Input: dimensioned drawing with shaded views. Units: mm. Origin: part minimum x, y, z. Round coordinates to 2 decimals unless told otherwise and drop trailing zeros. Write each loop counter-clockwise with the first axis right and the second up, starting at its lowest first coordinate (ties: lowest second). Pieces come first, ordered by that corner, then holes. Notation, with made-up numbers: (-23.5, -17) - (17.5, -17) arc R28 cw to (17.5, 11) - close; hole circle Ø8 at (27, 24). An arc over 180 degrees is marked (long way). Use one line per item in the form item = value.
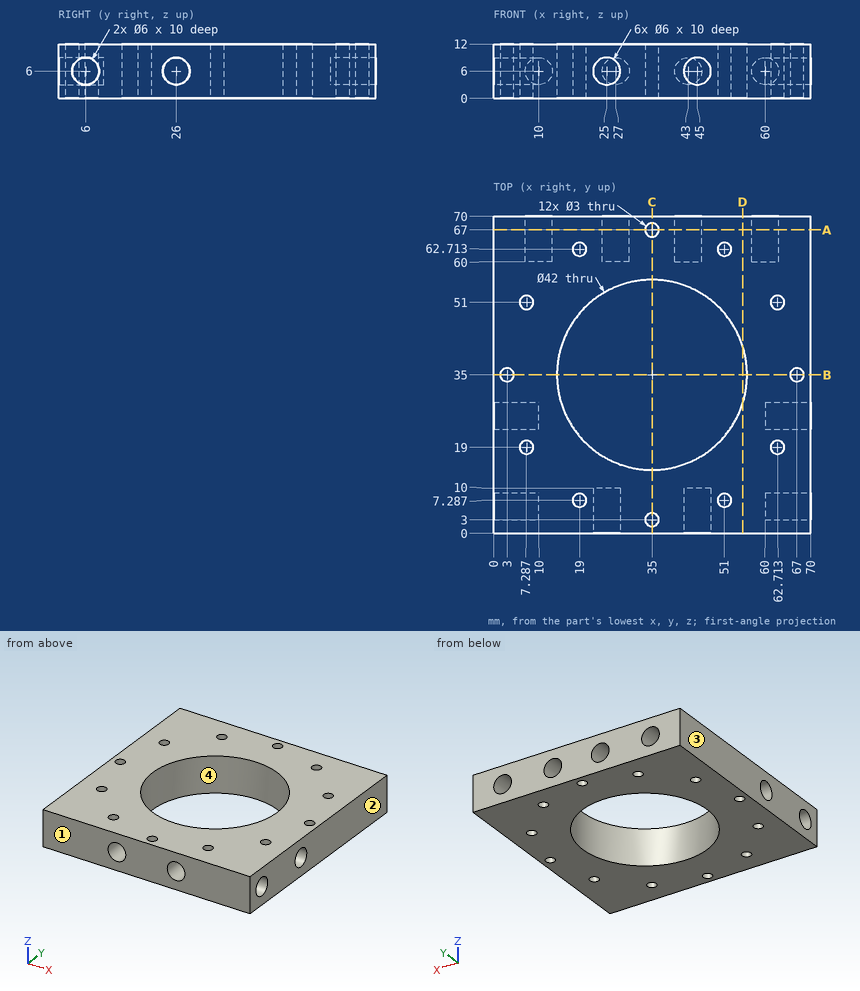
(1) Draft query along X for the marked faces 1, 2, 3 and 4. Return one class per face: released by +X, released by -X, zero draft, split by the parting line, or undercut.
Derived:
face_1 = zero draft
face_2 = released by +X
face_3 = released by -X
face_4 = undercut
(2) Cut plane D-D on x = 55. Output: boundary loops of the cut face in (y, z), then the cut area to 3 significant figures.
Derived:
outline = (0, 0) - (28.6, 0) - (28.6, 12) - (0, 12) - close; (41.4, 0) - (70, 0) - (70, 12) - (41.4, 12) - close
area = 686 mm^2
(3) Cut plane A-A on y = 67. Output: boundary loops of the cut face in (x, z), then the cut area to 3 significant figures.
Derived:
outline = (0, 0) - (33.5, 0) - (33.5, 12) - (0, 12) - close; (36.5, 0) - (70, 0) - (70, 12) - (36.5, 12) - close; hole circle Ø6 at (10, 6); hole circle Ø6 at (27, 6); hole circle Ø6 at (43, 6); hole circle Ø6 at (60, 6)
area = 691 mm^2
(4) Cut plane B-B on y = 35. Output: boundary loops of the cut face in (x, z), then the cut area to 3 significant figures.
Derived:
outline = (0, 0) - (1.5, 0) - (1.5, 12) - (0, 12) - close; (4.5, 0) - (14, 0) - (14, 12) - (4.5, 12) - close; (56, 0) - (65.5, 0) - (65.5, 12) - (56, 12) - close; (68.5, 0) - (70, 0) - (70, 12) - (68.5, 12) - close
area = 264 mm^2
(5) First-contact query: pin 1 Ø2.5 at (x, y) = (51, 7.29) entering from -Z; pin 2 Ø1.5 at (x, z) = (59, 7.5) entering from +Y; pin 3 Ø3 at (y, z) = (25, 7) entering from +X. Flat tips, straight axial feed; report the tip coordinate or a pass-through.
Derived:
pin_1 = through
pin_2 = 60
pin_3 = 60
(6) Material intervals for L1, parallel to X at y = 5.5, z = 5.75; L2, parallel to Y at x = 51, z = 9.25; L3, parallel to X at y = 67.25, z = 6, sorted ascending.
Derived:
L1 = 10 to 22.01, 27.99 to 42.01, 47.99 to 60
L2 = 0 to 5.79, 8.79 to 21.4, 48.6 to 61.21, 64.21 to 70
L3 = 0 to 7, 13 to 24, 30 to 33.52, 36.48 to 40, 46 to 57, 63 to 70
